Geometry check sheet. Reference: the model listing, model coordinates, mm. A direction names the side the tool comes from. Round coordinates to 2 decimals unless told otherwise and drop trailing zeros. Loops run counter-clockwise (first coordinate to the right, second up) from the corner with the lowest first, then second, coordinate; pieces in that order, holes last.
```python
from build123d import *

# Parameters (mm, degrees)
CYLINDER001_R     = 1.65
CYLINDER001_DEPTH = 30
ARRAY002_X_COUNT  = 2
ARRAY002_X_PITCH  = 13
ARRAY002_Y_COUNT  = 2
ARRAY002_Y_PITCH  = 53
CYLINDER003_R     = 0.9
CYLINDER003_DEPTH = 10
CYLINDER004_R     = 1.175
CYLINDER004_DEPTH = 10
CYLINDER005_R     = 1.5
CYLINDER005_DEPTH = 10
CYLINDER_R        = 1.65
CYLINDER_DEPTH    = 30
ARRAY001_X_COUNT  = 2
ARRAY001_X_PITCH  = 38
ARRAY001_Y_COUNT  = 3
ARRAY001_Y_PITCH  = 13
ARRAY_X_COUNT     = 3
ARRAY_X_PITCH     = 13
ARRAY_Y_COUNT     = 4
ARRAY_Y_PITCH     = 13
BOX_W             = 46
BOX_H             = 60
BOX_DEPTH         = 15


with BuildPart() as array002:
    # Cylinder001 → Cylinder001 (new body)
    with BuildSketch(Plane.XY.offset(-20)):
        Circle(CYLINDER001_R)
    extrude(amount=CYLINDER001_DEPTH)

    # Array002 X: Array002 ×2


with BuildPart() as array002_1:
    add(array002.part)
    with Locations(*[(i * ARRAY002_X_PITCH, 0, 0) for i in range(1, ARRAY002_X_COUNT)]):
        add(array002.part)

    # Array002 Y: Array002 ×2


with BuildPart() as array002_2:
    add(array002_1.part)
    with Locations(*[(0, i * ARRAY002_Y_PITCH, 0) for i in range(1, ARRAY002_Y_COUNT)]):
        add(array002_1.part)


with BuildPart() as array002_3:
    # Array002 placement: moved
    add(array002_2.part.moved(Location((16.5, 3.5, 0))))


with BuildPart() as cylinder003:
    # Cylinder003 → Cylinder003 (new body)
    with BuildSketch(Plane(origin=(30, 17, -9), x_dir=(1, 0, 0), z_dir=(0, 0, 1))):
        Circle(CYLINDER003_R)
    extrude(amount=CYLINDER003_DEPTH)


with BuildPart() as cylinder004:
    # Cylinder004 → Cylinder004 (new body)
    with BuildSketch(Plane(origin=(30, 43, -9), x_dir=(1, 0, 0), z_dir=(0, 0, 1))):
        Circle(CYLINDER004_R)
    extrude(amount=CYLINDER004_DEPTH)


with BuildPart() as cylinder005:
    # Cylinder005 → Cylinder005 (new body)
    with BuildSketch(Plane(origin=(16, 17, -9), x_dir=(1, 0, 0), z_dir=(0, 0, 1))):
        Circle(CYLINDER005_R)
    extrude(amount=CYLINDER005_DEPTH)


with BuildPart() as hole_union:
    # Cylinder → Cylinder (new body)
    with BuildSketch(Plane.XY.offset(-20)):
        Circle(CYLINDER_R)
    extrude(amount=CYLINDER_DEPTH)

    # Array001 X: hole union ×2


with BuildPart() as hole_union_1:
    add(hole_union.part)
    with Locations(*[(i * ARRAY001_X_PITCH, 0, 0) for i in range(1, ARRAY001_X_COUNT)]):
        add(hole_union.part)

    # Array001 Y: hole union ×3


with BuildPart() as hole_union_2:
    add(hole_union_1.part)
    with Locations(*[(0, i * ARRAY001_Y_PITCH, 0) for i in range(1, ARRAY001_Y_COUNT)]):
        add(hole_union_1.part)


with BuildPart() as hole_union_3:
    # Array001 placement: moved
    add(hole_union_2.part.moved(Location((4, 17, 0))))

    # Fusion001: union Array002, Cylinder003, Cylinder004, Cylinder005
    add(array002_3.part)
    add(cylinder003.part)
    add(cylinder004.part)
    add(cylinder005.part)


with BuildPart() as top_cone:
    # Cone → Cone (revolve)
    with BuildSketch(Plane(origin=(0, 0, -7), x_dir=(1, 0, 0), z_dir=(0, -1, 0))):
        Polygon((0, 0), (2.8, 0), (3, 7), (0, 7), align=None)
    revolve(axis=Axis((0, 0, -7), (0, 0, 1)))


with BuildPart() as cone_array:
    # Cone001 → Cone001 (revolve)
    with BuildSketch(Plane(origin=(0, 0, -19), x_dir=(-1, 0, 0), z_dir=(0, 1, 0))):
        Polygon((0, 0), (1.2, 0), (2.8, 12), (0, 12), align=None)
    revolve(axis=Axis((0, 0, -19), (0, 0, 1)))

    # Fusion: union top cone
    add(top_cone.part)


with BuildPart() as cone_array_1:
    # Fusion placement: moved
    add(cone_array.part.moved(Location((0, 0, 5))))

    # Array X: cone array ×3


with BuildPart() as cone_array_2:
    add(cone_array_1.part)
    with Locations(*[(i * ARRAY_X_PITCH, 0, 0) for i in range(1, ARRAY_X_COUNT)]):
        add(cone_array_1.part)

    # Array Y: cone array ×4


with BuildPart() as cone_array_3:
    add(cone_array_2.part)
    with Locations(*[(0, i * ARRAY_Y_PITCH, 0) for i in range(1, ARRAY_Y_COUNT)]):
        add(cone_array_2.part)


with BuildPart() as cone_array_4:
    # Array placement: moved
    add(cone_array_3.part.moved(Location((10, 10, 0))))


with BuildPart() as all_cut:
    # Box → Box (new body)
    with BuildSketch(Plane.XY.offset(-15)):
        with Locations((23, 30)):
            Rectangle(BOX_W, BOX_H)
    extrude(amount=BOX_DEPTH)

    # Cut: cut cone array
    add(cone_array_4.part, mode=Mode.SUBTRACT)

    # Cut001: cut hole union
    add(hole_union_3.part, mode=Mode.SUBTRACT)


solid = all_cut.part
```
1) Access from +Z, -Z, +X, -X, +Y, -Y to the whole of each face (thin tool, end or side, straight path). Record for faces 1 (the face through (10, 10, -14)), 2 (the face through (41.785, 31.636, -7.605)).
Report:
face 1: +Z
face 2: +Z, -Z
2) Sectioned sample at C-C, the plane z = -7. State how many separate pieces and enclosed holes the cut face has, then the cut area to 3 significant figures.
Report:
separate pieces: 1
enclosed holes: 25
area: 2,490 mm2
3) Sectioned sample at A-A, the plane y = 43. Record the cut outline in (x, z) (3 decimals).
Report:
outline: (0, -15) - (2.35, -15) - (2.35, 0) - (0, 0) - close; (5.65, -15) - (40.35, -15) - (40.35, 0) - (31.175, 0) - (31.175, -9) - (28.825, -9) - (28.825, 0) - (5.65, 0) - close; (43.65, -15) - (46, -15) - (46, 0) - (43.65, 0) - close
4) Scan lines: line 1 along Y through (x, z) = (4, -1.5); line 2 along X through (y, z) = (43, -13); line 3 along X through (y, z) = (43, -3.75) (3 decimals). Record each from-to range of solid material in increasing order.
Report:
line 1: y = 0 to 15.35, 18.65 to 28.35, 31.65 to 41.35, 44.65 to 60
line 2: x = 0 to 2.35, 5.65 to 40.35, 43.65 to 46
line 3: x = 0 to 2.35, 5.65 to 28.825, 31.175 to 40.35, 43.65 to 46
5) Gauge pin test, flat ends, axial feed: pin 1 (2 mm diameter, centred on x = 42, y = 43, fed in from +Z); pin 2 (0.7 mm diameter, centred on x = 35.5, y = 48.5, fed in from +Z); pin 3 (0.7 mm diameter, centred on x = 30.5, y = 42.5, fed in from +Z). Record the tip position at first contact, or that the pin passes through.
Report:
pin 1: passes through
pin 2: stops at z = -14
pin 3: stops at z = -9
6) Sectioned sample at B-B, the plane x = 4. Record the cut outline in (y, z).
Report:
outline: (0, -15) - (15.35, -15) - (15.35, 0) - (0, 0) - close; (18.65, -15) - (28.35, -15) - (28.35, 0) - (18.65, 0) - close; (31.65, -15) - (41.35, -15) - (41.35, 0) - (31.65, 0) - close; (44.65, -15) - (60, -15) - (60, 0) - (44.65, 0) - close
7) Sectioned sample at D-D, the plane x = 30. Record the cut outline in (y, z) (3 decimals).
Report:
outline: (0, -15) - (1.928, -15) - (1.928, 0) - (0, 0) - close; (5.072, -15) - (54.928, -15) - (54.928, 0) - (44.175, 0) - (44.175, -9) - (41.825, -9) - (41.825, 0) - (17.9, 0) - (17.9, -9) - (16.1, -9) - (16.1, 0) - (5.072, 0) - close; (58.072, -15) - (60, -15) - (60, 0) - (58.072, 0) - close
